For this review, take the finished solid that the model builds, in its own axes (mm). Face numbers are marked on the shaded views. A direction names the side the tool comes from. Coordinates: 2 decimals unless noted, no trailing zeros. Order: outer loops, then holes, each group sorted by start corner. A loop starts at its lowest first (then second) coordinate and runs counter-clockwise, first axis right, second up. Notation, with made-up numbers: (72.5, 4.25) -> (110.5, 4.25) arc R32 ccw to (110.5, 30.25) -> close; hole circle Ø2 at (1.5, 47). An arc over 180 degrees is marked (long way). Answer as a JSON object with one key per item and string values. Group by question number.
1) Add section B-B, the plane x = 289.5. Write out the cut boundary in (y, z), then the cut area to 3 significant figures.
2) Draft analysis for pull direction Z (two halves, no side actions). For the marked faces 3 and 4, state which applies: +Z half, -Z half, draft (parallel to the pull), parting line (faces both ways), or undercut.
3) Machinability: for the marked faces 1 and 2, which of the approach directions +Z, -Z, +X, -X, +Y, -Y give a long, thin tool a straight path to every point of the face, cutting with its end or side? Answer none if there is none.
4) Add section A-A, the plane x = 4.5. Write out the cut boundary in (y, z).
5) Wall thickness on L1, parallel to Y at x = -193.5, z = 0; L2, parallel to Y at x = 65.5, z = -9; L3, parallel to Z at x = -70, y = -15: over which ranges is each line inside the solid? List them lowest first.
6) For pin 1 (10 mm diameter, centred on x = -252, y = -7.5, fed in from +Z); pin 2 (8 mm diameter, centred on x = -126.5, z = 6.5, fed in from -Y); pin 3 (5 mm diameter, centred on x = 45, z = 10, fed in from +Y), all flat-tipped, find the tip position at first contact; note any pin that passes through.
from build123d import *

# Parameters (mm, degrees)
KES_EKSTR_ZYON1_DEPTH = 431
KES_EKSTR_ZYON2_DEPTH = 4


with BuildPart() as part:
    # Çizim1 → Döndür1 (revolve)
    with BuildSketch(Plane.XY):
        Polygon((-330.5, 0), (330.5, 0), (330.5, 15), (210.5, 15), (210.5, 17.5), (-220.5, 17.5), (-220.5, 15), (-330.5, 15), align=None)
    revolve(axis=Axis((-330.5, 0, 0), (1, 0, 0)))

    # Çizim2 → Kes-Ekstrüzyon1 (cut)
    with BuildSketch(Plane.ZY.offset(220.5)):
        with BuildLine():
            Line((-15, 9.013878189), (-15, -9.013878189))
            ThreePointArc((-15, -9.013878189), (-17.5, 0), (-15, 9.013878189))
        make_face()
        with BuildLine():
            Line((15, 9.013878189), (15, -9.013878189))
            ThreePointArc((15, -9.013878189), (17.5, 0), (15, 9.013878189))
        make_face()
    extrude(amount=-KES_EKSTR_ZYON1_DEPTH, mode=Mode.SUBTRACT)

    # Çizim3 → Kes-Ekstrüzyon2 (cut)
    with BuildSketch(Plane(origin=(0, 15, 0), x_dir=(1, 0, 0), z_dir=(0, 1, 0))):
        with BuildLine():
            Line((324.5, -4), (299.5, -4))
            ThreePointArc((299.5, -4), (295.5, 0), (299.5, 4))
            Line((299.5, 4), (324.5, 4))
            ThreePointArc((324.5, 4), (328.5, 0), (324.5, -4))
        make_face()
    extrude(amount=-KES_EKSTR_ZYON2_DEPTH, mode=Mode.SUBTRACT)


solid = part.part
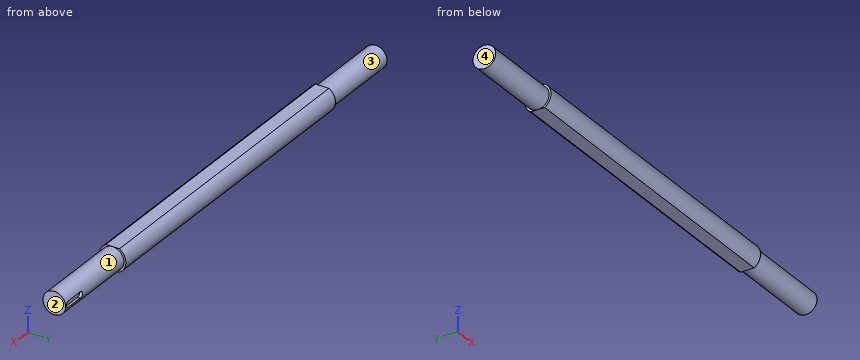
Output values:
{
 "1": {"outline": "circle Ø30 at (0, 0)", "area": "707 mm²"},
 "2": {"face 3": "parting line", "face 4": "draft"},
 "3": {"face 1": "+X", "face 2": "+Z, -Z, +X, +Y, -Y"},
 "4": {"outline": "(-9.01, -15) -> (9.01, -15) arc R17.5 ccw to (9.01, 15) -> (-9.01, 15) arc R17.5 ccw to start"},
 "5": {"L1": "y = -17.5 to 17.5", "L2": "y = -15.01 to 15.01", "L3": "z = -9.01 to 9.01"},
 "6": {"pin 1": "stops at z = 14.79", "pin 2": "stops at y = -17.32", "pin 3": "stops at y = 15.81"}
}
